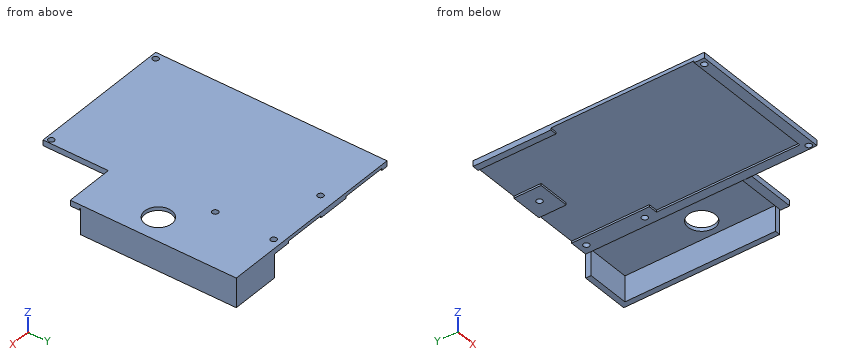
Autodesk Inventor part; units mm, degrees
ref_plane "Work Plane2" through (26.5, 18.8696, -13.1) normal (0, 0, 1) x (1, 0, 0)
ref_plane "YZ Plane" through (0, 0, 0) normal (1, 0, 0) x (0, 1, 0)
ref_plane "XZ Plane" through (0, 0, 0) normal (0, 1, 0) x (-1, 0, 0)
ref_plane "Work Plane1" through (0, 0, 0) normal (0, 0, 1) x (1, 0, 0)
sketch "Sketch1" plane through (0, 0, 0) normal (0, 0, 1) x (1, 0, 0)
  circle A0 centre (-49.8552, -60.9647) radius 1.65 construction
  circle A1 centre (24.2311, -60.9647) radius 1.65 construction
  arc A2 (22.7622, -32.9022) -> (21.5, -36.5843) centre (37.7579, -40.1) ccw construction
  line L0 (22.7622, -32.9022) -> (25.7, -32.9022) construction
  line L1 (25.7, -32.9022) -> (25.7, -35.65) construction
  arc A3 (25.7, -44.55) -> (25.7, -35.65) centre (2.4892, -40.1) ccw construction
  line L2 (25.7, -44.55) -> (25.7, -47.2978) construction
  line L3 (25.7, -47.2978) -> (22.7622, -47.2978) construction
  arc A4 (21.5, -43.6157) -> (22.7622, -47.2978) centre (37.7579, -40.1) ccw construction
  line L4 (21.5, -58.1715) -> (21.5, -43.6157) construction
  line L5 (-53.5, -58.1715) -> (21.5, -58.1715) construction
  line L6 (-53.5, -63.7578) -> (-53.5, -58.1715) construction
  line L7 (26.5, -63.7578) -> (-53.5, -63.7578) construction
  line L8 (26.5, -27.7578) -> (26.5, -63.7578) construction
  line L9 (53.5, -27.7578) -> (26.5, -27.7578) construction
  line L10 (53.5, -22.7578) -> (53.5, -27.7578) construction
  line L11 (21.5, -22.7578) -> (53.5, -22.7578) construction
  line L12 (21.5, -36.5843) -> (21.5, -22.7578) construction
  line L13 (21.5, -39.9422) -> (21.5, 19.8578) construction
  line L14 (26.5, 63.7578) -> (26.5, 13.7578) construction
  line L15 (16.5, 20.8578) -> (16.5, 63.7578) construction
  line L16 (-6.7098, 63.7578) -> (-6.7098, 48.6857) construction
  line L17 (-24.537, 20.8578) -> (-24.537, 63.7578) construction
  line L18 (-49.8552, 63.7578) -> (-49.8552, 20.8578) construction
  line L19 (-53.5, 63.7578) -> (-53.5, -63.7578) construction
  line L20 (-53.5, -63.7578) -> (26.5, -63.7578)
  line L21 (26.5, -63.7578) -> (26.5, -58.1715)
  line L22 (26.5, -58.1715) -> (-53.5, -58.1715)
  line L23 (-53.5, -58.1715) -> (-53.5, -63.7578)
  line L24 (21.5, -58.1715) -> (26.5, -58.1715)
  line L25 (26.5, -58.1715) -> (26.5, 20.8578)
  line L26 (26.5, 20.8578) -> (21.5, 20.8578)
  line L27 (21.5, 20.8578) -> (21.5, -58.1715)
  line L28 (16.5, 20.8578) -> (26.5, 20.8578)
  line L29 (26.5, 20.8578) -> (26.5, 63.7578)
  line L30 (26.5, 63.7578) -> (16.5, 63.7578)
  line L31 (16.5, 63.7578) -> (16.5, 20.8578)
  line L32 (-49.8552, 63.7578) -> (-24.537, 63.7578)
  line L33 (-24.537, 63.7578) -> (-24.537, 20.8578)
  line L34 (-24.537, 20.8578) -> (-49.8552, 20.8578)
  line L35 (-49.8552, 20.8578) -> (-49.8552, 63.7578)
  line L36 (26.6067, -27.7578) -> (53.5, -27.7578)
  line L37 (53.5, -27.7578) -> (53.5, -22.7578)
  line L38 (53.5, -22.7578) -> (26.6067, -22.7578)
  line L39 (26.6067, -22.7578) -> (26.6067, -27.7578)
  line L40 (-6.7098, 63.7578) -> (-24.537, 63.7578)
  line L41 (-24.537, 63.7578) -> (-24.537, 48.6857)
  line L42 (-24.537, 48.6857) -> (-6.7098, 48.6857)
  line L43 (-6.7098, 48.6857) -> (-6.7098, 63.7578)
  circle A5 centre (21.5, 59.4877) radius 1.65
  circle A6 centre (24.2311, -60.9647) radius 1.65
  circle A7 centre (-49.8552, -60.9647) radius 1.65
  circle A8 centre (-16, 56.2217) radius 1.65
  line L44 (-53.5, 63.7578) -> (-49.8552, 63.7578)
  line L45 (-49.8552, 63.7578) -> (-49.8552, 20.8578)
  line L46 (-49.8552, 20.8578) -> (-53.5, 20.8578)
  line L47 (-53.5, 20.8578) -> (-53.5, 63.7578)
  circle A9 centre (21.5, 27.3048) radius 1.65
  point P0 (0, 0)
extrude "Extrusion1" add sketch "Sketch1" along normal blind 1.1 contours L23 L22 L21 L20 | L22 L27 L26 L25 | L26 L28 L31 L30 L29 | L35 L46 L47 L44 | L40 L43 L42 L33 | L39 L38 L37 L36
sketch "Sketch2" plane through (0, 0, 1.1) normal (0, 0, 1) x (1, 0, 0)
  circle A0 centre (-49.8552, -60.9647) radius 1.65
  circle A1 centre (24.2311, -60.9647) radius 1.65
  circle A2 centre (21.5, 59.4877) radius 1.65
  line L0 (26.5, -63.7578) -> (26.5, 63.7578)
  line L1 (26.5, 63.7578) -> (16.5, 63.7578)
  line L2 (16.5, 63.7578) -> (16.5, 20.8578)
  line L3 (16.5, 20.8578) -> (21.5, 20.8578)
  line L4 (21.5, 20.8578) -> (21.5, -58.1715)
  line L5 (21.5, -58.1715) -> (-53.5, -58.1715)
  line L6 (-53.5, -58.1715) -> (-53.5, -63.7578)
  line L7 (-53.5, -63.7578) -> (26.5, -63.7578)
  line L8 (-49.8552, 63.7578) -> (-49.8552, 20.8578)
  line L9 (-6.7098, 63.7578) -> (-49.8552, 63.7578)
  line L10 (21.5, 20.8578) -> (16.5, 20.8578)
  line L11 (-49.8552, 63.7578) -> (16.5, 63.7578)
  line L12 (16.5, 63.7578) -> (16.5, 20.8578)
  line L13 (16.5, 20.8578) -> (-49.8552, 20.8578)
  line L14 (-49.8552, 20.8578) -> (-49.8552, 63.7578)
  line L15 (21.5, -58.1715) -> (-53.5, -58.1715)
  line L16 (-49.8552, 20.8578) -> (21.5, 20.8578)
  line L17 (21.5, 20.8578) -> (21.5, -58.1715)
  line L18 (21.5, -58.1715) -> (-49.8552, -58.1715)
  line L19 (-49.8552, -58.1715) -> (-49.8552, 20.8578)
  line L20 (-53.5, -58.1715) -> (-49.8552, -58.1715)
  line L21 (-49.8552, -58.1715) -> (-49.8552, 63.7578)
  line L22 (-49.8552, 63.7578) -> (-53.5, 63.7578)
  line L23 (-53.5, 63.7578) -> (-53.5, -58.1715)
  line L24 (53.5, -27.7578) -> (53.5, -22.7578)
  line L25 (26.5, 63.7578) -> (53.5, 63.7578)
  line L26 (53.5, 63.7578) -> (53.5, -27.7578)
  line L27 (53.5, -27.7578) -> (26.5, -27.7578)
  line L28 (26.5, -27.7578) -> (26.5, 63.7578)
  circle A3 centre (21.5, 59.4877) radius 1.65
  circle A4 centre (-16, 56.2217) radius 1.65
  line L29 (16.5, 63.7578) -> (16.5, 20.8578)
  line L30 (16.5, 63.7578) -> (26.5, 63.7578)
  circle A5 centre (24.2311, -60.9647) radius 1.65
  line L31 (16.5, 20.8578) -> (-49.8552, 20.8578)
  line L32 (-49.8552, 20.8578) -> (-49.8552, 63.7578)
  line L33 (-49.8552, 63.7578) -> (16.5, 63.7578)
  line L34 (16.5, 63.7578) -> (16.5, 20.8578)
  ellipse E0 centre (39.7, 10.0578) end of major axis (44.7, 10.0578) minor radius 3.5355
  circle A6 centre (39.7, 10.0578) radius 7.5
  circle A7 centre (21.5, 27.3048) radius 1.65
  point P0 (0, 0)
  dimension "d4" = 15
extrude "Extrusion2" add sketch "Sketch2" along normal blind 2 contours L7 L6 L5 L4 L3 L2 L1 L0 | L0 L25 L26 L24 L27 | L23 L22 L8 L19 L5 | L2 L13 L8 L9 L11 | L19 L13 L3 L4 L5
ref_plane "Work Plane2" through (26.5, 18.8696, -13.1) normal (0, 0, 1) x (1, 0, 0)
sketch "Sketch3" plane through (0, 0, 1.1) normal (0, 0, -1) x (-1, 0, 0)
  circle A0 centre (16, 56.2217) radius 1.65
  circle A1 centre (-39.7, 10.0578) radius 7.5
  circle A2 centre (-21.5, 59.4877) radius 1.65
  circle A3 centre (-24.2311, -60.9647) radius 1.65
  circle A4 centre (49.8552, -60.9647) radius 1.65
  line L0 (-53.5, 63.7578) -> (53.5, 63.7578)
  line L1 (53.5, 63.7578) -> (53.5, -63.7578)
  line L2 (53.5, -63.7578) -> (-26.5, -63.7578)
  line L3 (-26.5, -63.7578) -> (-26.5, -27.7578)
  line L4 (-26.5, -27.7578) -> (-53.5, -27.7578)
  line L5 (-53.5, -27.7578) -> (-53.5, 63.7578)
  line L6 (-26.5, 18.8696) -> (-45, 18.8696)
  line L7 (-45, 18.8696) -> (-45, 63.7578)
  line L8 (-45, 63.7578) -> (-26.5, 63.7578)
  line L9 (-26.5, 63.7578) -> (-26.5, 18.8696)
  line L10 (-70.915, -41.1304) -> (-130.915, -41.1304)
  line L11 (-130.915, -41.1304) -> (-130.915, 18.8696)
  line L12 (-130.915, 18.8696) -> (-45, 18.8696)
  line L13 (-45, 18.8696) -> (-45, 5.872)
  line L14 (-45, 5.872) -> (-26.5, 5.872)
  line L15 (-26.5, 5.872) -> (-26.5, 13.7578)
  line L16 (-26.5, 13.7578) -> (-21.5, 13.7578)
  line L17 (-21.5, 13.7578) -> (-21.5, 19.8578)
  line L18 (-21.5, 19.8578) -> (53.5, 19.8578)
  line L19 (53.5, 19.8578) -> (53.5, -58.1715)
  line L20 (53.5, -58.1715) -> (-21.5, -58.1715)
  line L21 (-21.5, -58.1715) -> (-21.5, -39.9578)
  line L22 (-21.5, -39.9578) -> (-21.5, -22.7578)
  line L23 (-21.5, -22.7578) -> (-28.8534, -22.7578)
  line L24 (-28.8534, -22.7578) -> (-28.8534, -2.7892)
  line L25 (-28.8534, -2.7892) -> (-50.0866, -2.7892)
  line L26 (-50.0866, -2.7892) -> (-50.0866, -22.7578)
  line L27 (-50.0866, -22.7578) -> (-53.5, -22.7578)
  line L28 (-53.5, -22.7578) -> (-53.5, -27.7578)
  line L29 (-53.5, -27.7578) -> (-70.915, -27.7578)
  line L30 (-70.915, -27.7578) -> (-70.915, -41.1304)
  circle A5 centre (-125.915, -11.1304) radius 2.95
  circle A6 centre (-125.915, -36.1304) radius 2.95
  circle A7 centre (-100.915, -36.1304) radius 2.95
  circle A8 centre (-75.915, -36.1304) radius 2.95
  circle A9 centre (-75.915, -11.1304) radius 2.95
  circle A10 centre (-75.915, 13.8696) radius 2.95
  circle A11 centre (-100.915, 13.8696) radius 2.95
  circle A12 centre (-125.915, 13.8696) radius 2.95
  line L31 (-53.5, 63.7578) -> (53.5, 63.7578)
  line L32 (-53.5, 63.7578) -> (-50.5, 63.7578)
  line L33 (-50.5, 63.7578) -> (-50.5, -22.2422)
  line L34 (-50.5, -22.2422) -> (-53.5, -22.2422)
  line L35 (-53.5, -22.2422) -> (-53.5, 63.7578)
  line L36 (-50.5, 63.7578) -> (-26.5, 63.7578)
  line L37 (-26.5, 63.7578) -> (-26.5, 60.7578)
  line L38 (-26.5, 60.7578) -> (-50.5, 60.7578)
  line L39 (-50.5, 60.7578) -> (-50.5, 63.7578)
  line L40 (-16.5, 63.7578) -> (-26.5, 63.7578)
  line L41 (-50.5, 60.7578) -> (-26.5, 60.7578)
  line L42 (-26.5, 60.7578) -> (-26.5, 63.7578)
  line L43 (-26.5, 63.7578) -> (-50.5, 63.7578)
  line L44 (-50.5, 63.7578) -> (-50.5, 60.7578)
  point P0 (0, 0)
  dimension "d5" = 3
  dimension "d6" = 86
  dimension "d7" = 3
extrude "Extrusion3" add sketch "Sketch3" along normal up to surface (14.2 mm away) contours L38 L33 L0 L7 | L7 L0 L9 L38 | L33 L34 L5 L12 | L12 L5 L0 L33
properties part number "10_MiniSPIM_Lid"
Input: part model. Units: mm. Frame: model coordinates. Coordinates: 2 decimals unless noted, no trailing zeros. Loops run counter-clockwise (first coordinate to the right, second up) from the corner with the lowest first, then second, coordinate; pieces in that order, holes last. Notation, with made-up numbers: (-4.5, -1.75) - (54.5, -1.75) arc R14 ccw to (54.5, 7.25) - close; hole circle Ø7 at (19.25, 3.25). An arc over 180 degrees is marked (long way). Answer in a Markdown table with one row per item. Add a question column.
Item 1: Section query B-B on y = 34.5. Return the cut outline in (x, z), then the cut area to 3 significant figures.
Item 2: Line query: line 1 along Y through (x, z) = (39.7, 2.65); line 2 along Y through (x, z) = (21.5, 1.3); line 3 along Z through (x, y) = (8, 35). Output: solid intervals per line, ascending. Write a range as [from, to].
Item 3: Section query A-A on x = 39.7. Return the cut outline in (y, z).
Item 4: Contact query for flat-ended pins moving along their axis: P1, Ø5, axis at x = 34, z = -1.5, coming from the -Y side; P2, Ø3, axis at x = 24.23, y = -60.96, coming from the +Z side; P3, Ø3, axis at y = 17.5, z = -3, coming from the -X side; P4, Ø3, axis at x = -32.5, y = 37, coming from the -Z side. Output: stop coordinate, or through.
Item 5: Section query D-D on y = 8.5. Return the cut outline in (x, z).
Item 6: Section query C-C on x = -21. Return the cut outline in (y, z), then the cut area to 3 significant figures.
Recorded:
| question | item | result |
|---|---|---|
| 1 | outline | (-53.5, 0) - (-49.86, 0) - (-49.86, 1.1) - (16.5, 1.1) - (16.5, 0) - (26.5, 0) - (26.5, 1.1) - (50.5, 1.1) - (50.5, -13.1) - (53.5, -13.1) - (53.5, 3.1) - (-53.5, 3.1) - close |
| 1 | area | 272 mm^2 |
| 2 | line 1 | [-27.76, 2.56], [17.56, 63.76] |
| 2 | line 2 | [-63.76, 25.65], [28.95, 57.84], [61.14, 63.76] |
| 2 | line 3 | [1.1, 3.1] |
| 3 | outline | (-27.76, 0) - (-22.76, 0) - (-22.76, 1.1) - (2.56, 1.1) - (2.56, 3.1) - (-27.76, 3.1) - close; (17.56, 1.1) - (60.76, 1.1) - (60.76, -13.1) - (63.76, -13.1) - (63.76, 3.1) - (17.56, 3.1) - close |
| 4 | P1 | y = -27.76 |
| 4 | P2 | through |
| 4 | P3 | x = 50.5 |
| 4 | P4 | z = 1.1 |
| 5 | outline | (-53.5, 1.1) - (21.5, 1.1) - (21.5, 0) - (26.5, 0) - (26.5, 1.1) - (32.36, 1.1) - (32.36, 3.1) - (-53.5, 3.1) - close; (47.04, 1.1) - (50.5, 1.1) - (50.5, -13.1) - (53.5, -13.1) - (53.5, 3.1) - (47.04, 3.1) - close |
| 6 | outline | (-63.76, 0) - (-58.17, 0) - (-58.17, 1.1) - (48.69, 1.1) - (48.69, 0) - (63.76, 0) - (63.76, 3.1) - (-63.76, 3.1) - close |
| 6 | area | 278 mm^2 |
